Autodesk Inventor part; units mm, degrees
ref_plane "Work Plane1" through (0, -32, 0) normal (0, 1, 0) x (-1, 0, 0)
ref_plane "Work Plane2" through (0, 10, 0) normal (0, 1, 0) x (-1, 0, 0)
ref_plane "YZ Plane" through (0, 0, 0) normal (1, 0, 0) x (0, 1, 0)
sketch "Sketch1" plane through (0, 0, 0) normal (0, 0, 1) x (1, 0, 0)
  line L0 (-16.45, 0) -> (38.85, 0)
  line L1 (0, -84.7) -> (0, 23.1)
  line L2 (-12.5, -29.4576) -> (-12.5, -21.4576)
  line L3 (-12.5, -21.4576) -> (12.5, -21.4576)
  line L4 (12.5, -21.4576) -> (12.5, -29.4576)
  arc A0 (-12.5, -29.4576) -> (12.5, -29.4576) centre (0, 0) ccw
  arc A1 (0, -77) -> (0, -23) centre (0, -50) ccw
  line L5 (0, -77) -> (0, -23)
  dimension "d0" = 32
  dimension "d1" = 8
  dimension "d2" = 25
  dimension "d5" = 27
  dimension "d6" = 50
extrude "Extrusion1" add sketch "Sketch1" along normal mid plane 13 contours A0 L2 L3 L1 | L1 A1 L4 A0 | A1 L1 L3 L4 picked at (1.4378, -26.1156)
revolve "Revolution1" cut sketch "Sketch1" angle 360 about axis through (0, -10, 0) along (0, 1, 0) keep common part contours L1 A0 L4 A1 | L1 A1 L4 A0
ref_plane "Work Plane1" through (0, -32, 0) normal (0, 1, 0) x (-1, 0, 0)
ref_plane "Work Plane2" through (0, 10, 0) normal (0, 1, 0) x (-1, 0, 0)
sketch "Sketch2" plane through (0, 10, 0) normal (0, 1, 0) x (-1, 0, 0)
  circle A0 centre (0, 0) radius 6.5
  line L0 (-12.5, 6.5) -> (12.5, 6.5)
extrude "Extrusion2" add sketch "Sketch2" against normal up to next
sketch "Sketch3" plane through (0, 0, 0) normal (1, 0, 0) x (0, 1, 0)
  line L0 (1.2, 0) -> (12.4, 0)
  circle A0 centre (4, 0) radius 2
  line L1 (10, 6.5) -> (10, -6.5)
  dimension "d11" = 4
  dimension "d12" = 6
extrude "Extrusion3" cut sketch "Sketch3" along normal through all both and the other way through all
properties part number "Stem" material "Bronze, Soft Tin"
Source: CAD feature listing. Evaluate the final solid. Frame: model axes, mm. A direction names the side the tool comes from. Round coordinates to 2 decimals unless told otherwise and drop trailing zeros. Order: outer loops, then holes, each group sorted by start corner. A loop starts at its lowest first (then second) coordinate and runs counter-clockwise, first axis right, second up. Notation, with made-up numbers: (59.25, 68) - (114.25, 68) arc R13 ccw to (114.25, 81) - close; hole circle Ø2 at (-40, 35). An arc over 180 degrees is marked (long way). Use a Markdown table: item, result. Add a question column.
1. Section query A-A (z = 0). Return the cut outline in (x, y).
2. Mould query, pull axis Y, two halves, no side actions, for faces 1 (the cylindrical face through (0, -32, 0)), 2 (the flat face through (0, -28, 6.5)), 3 (the cylindrical face through (0.1, 2.4, -1.2)). Classes: +Y half, -Y half, draft (parallel to the pull), parting line (faces both ways), or undercut.
3. First-contact query: pin 1 (5 mm diameter, centred on x = 5, z = 3.5, fed in from -Y); pin 2 (6.5 mm diameter, centred on y = 4, z = 0, fed in from -X); pin 3 (5 mm diameter, centred on y = 3.5, z = -3.5, fed in from -X). Flat tips, straight axial feed; report the tip coordinate or a pass-through.
4. Set-up query: faces 4 (the flat face through (-12.5, -28, 0)), 5 (the cylindrical face through (-6.2, -6.66, 1.95)). Return all of +Z, -Z, +X, -X, +Y, -Y with unobstructed straight access to the full face (end or side cutting, diameter ignored); none if empty.
5. Section query C-C (z = -4.5). Return the cut outline in (x, y).
6. Section query B-B (x = -4.5). Return the cut outline in (y, z).
7. Line query: probe 1 along Y at (x, z) = (-0.5, 0); probe 2 along Z at (x, y) = (3, 5); probe 3 along Z at (x, y) = (-1, 4). Output: solid intervals per line, ascending.
8. Section query D-D (y = 4). Return the cut outline in (x, z), then the cut area to 3 significant figures.
Derived:
| question | item | result |
|---|---|---|
| 1 | outline | (-12.5, -29.46) arc R32 ccw to (12.5, -29.46) - (12.5, -26.07) arc R27 ccw to (6.5, -23.79) - (6.5, 2) - (-6.5, 2) - (-6.5, -23.79) arc R27 ccw to (-12.5, -26.07) - close; (-6.5, 6) - (6.5, 6) - (6.5, 10) - (-6.5, 10) - close |
| 2 | face 1 | -Y half |
| 2 | face 2 | draft |
| 2 | face 3 | undercut |
| 3 | pin 1 | y = -31.9 |
| 3 | pin 2 | x = -6.5 |
| 3 | pin 3 | x = -6.38 |
| 4 | face 4 | +Z, -Z, -X, +Y, -Y |
| 4 | face 5 | +Y |
| 5 | outline | (-12.5, -29.46) arc R32 ccw to (12.5, -29.46) - (12.5, -26.49) arc R26.62 ccw to (4.69, -23.79) - (4.69, 10) - (-4.69, 10) - (-4.69, -23.79) arc R26.62 ccw to (-12.5, -26.49) - close |
| 6 | outline | (-31.68, -6.5) - (-24.18, -6.5) arc R26.62 ccw to (-23.79, -4.69) - (10, -4.69) - (10, 4.69) - (-23.79, 4.69) arc R26.62 ccw to (-24.18, 6.5) - (-31.68, 6.5) - close; hole circle Ø4 at (4, 0) |
| 7 | probe 1 | -32 to 2, 6 to 10 |
| 7 | probe 2 | -5.77 to -1.73, 1.73 to 5.77 |
| 7 | probe 3 | -6.42 to -2, 2 to 6.42 |
| 8 | outline | (-6.18, -2) arc R6.5 ccw to (6.18, -2) - close; (-6.18, 2) - (6.18, 2) arc R6.5 ccw to start |
| 8 | area | 81.6 mm2 |
